```python
from build123d import *

# Parameters (mm, degrees)
F0_R     = 1.9812
F0_R_2   = 1.5
F0_R_3   = 1.3716
F0_W     = 4.99999
F0_H     = 51.988198
F0_W_2   = 17
F0_H_2   = 10.000005
F1_DEPTH = 2.999994


with BuildPart() as f1:
    # F0 (on Top) → F1 (new body)
    with BuildSketch(Plane.XY):
        with BuildLine():
            ThreePointArc((-161.572698, -117.981502), (-160.412138, -120.783342), (-157.610298, -121.943902))
            Line((-157.610298, -121.943902), (139.264902, -121.943902))
            Line((139.264902, -121.943902), (219.265302, -121.943902))
            ThreePointArc((219.265302, -121.943902), (222.066859, -120.783459), (223.227302, -117.981902))
            Line((223.227302, -117.981902), (223.227302, 117.807098))
            ThreePointArc((223.227302, 117.807098), (222.066859, 120.608655), (219.265302, 121.769098))
            Line((219.265302, 121.769098), (143.227302, 121.769098))
            Line((143.227302, 121.769098), (-9.640698, 121.769098))
            ThreePointArc((-9.640698, 121.769098), (-12.442255, 120.608655), (-13.602698, 117.807098))
            Line((-13.602698, 117.807098), (-13.602698, 113.769098))
            Line((-13.602698, 113.769098), (-18.621498, 113.769098))
            Line((-18.621498, 113.769098), (-18.621498, 111.609098))
            ThreePointArc((-18.621498, 111.609098), (-20.602698, 109.627898), (-22.583898, 111.609098))
            Line((-22.583898, 111.609098), (-22.583898, 113.769098))
            Line((-22.583898, 113.769098), (-143.081498, 113.769098))
            Line((-143.081498, 113.769098), (-143.081498, 111.609098))
            ThreePointArc((-143.081498, 111.609098), (-145.062698, 109.627898), (-147.043898, 111.609098))
            Line((-147.043898, 111.609098), (-147.043898, 113.769098))
            Line((-147.043898, 113.769098), (-157.610698, 113.769098))
            ThreePointArc((-157.610698, 113.769098), (-160.412255, 112.608655), (-161.572698, 109.807098))
            Line((-161.572698, 109.807098), (-161.572698, -117.981502))
        make_face()
        with Locations((-145.062698, -115.720902)):
            Circle(F0_R, mode=Mode.SUBTRACT)
        with Locations((-156.572698, -110.230902)):
            Circle(F0_R_2, mode=Mode.SUBTRACT)
        with Locations((-99.431735, -91.208814)):
            Circle(F0_R_3, mode=Mode.SUBTRACT)
        with Locations((-20.602698, -115.720902)):
            Circle(F0_R, mode=Mode.SUBTRACT)
        with Locations((30.427302, -110.230902)):
            Circle(F0_R_2, mode=Mode.SUBTRACT)
        with Locations((-50.435135, -91.208814)):
            Circle(F0_R_3, mode=Mode.SUBTRACT)
        with Locations((-43.882665, -62.214709)):
            Rectangle(F0_W, F0_H, mode=Mode.SUBTRACT)
        with Locations((20.768265, -91.208814)):
            Circle(F0_R_3, mode=Mode.SUBTRACT)
        with Locations((-145.062698, -43.330902)):
            Circle(F0_R, mode=Mode.SUBTRACT)
        with Locations((-99.431735, -33.220614)):
            Circle(F0_R_3, mode=Mode.SUBTRACT)
        with Locations((-156.572698, -4.230902)):
            Circle(F0_R_2, mode=Mode.SUBTRACT)
        with Locations((-93.072694, -24.711481)):
            Rectangle(F0_W_2, F0_H_2, mode=Mode.SUBTRACT)
        with Locations((-50.435135, -33.220614)):
            Circle(F0_R_3, mode=Mode.SUBTRACT)
        with Locations((-20.602698, -43.330902)):
            Circle(F0_R, mode=Mode.SUBTRACT)
        with Locations((20.768265, -33.220614)):
            Circle(F0_R_3, mode=Mode.SUBTRACT)
        with Locations((27.127306, -24.711481)):
            Rectangle(F0_W_2, F0_H_2, mode=Mode.SUBTRACT)
        with Locations((-6.572698, -4.230902)):
            Circle(F0_R_2, mode=Mode.SUBTRACT)
        with Locations((69.764865, -91.208814)):
            Circle(F0_R_3, mode=Mode.SUBTRACT)
        with Locations((76.317335, -62.214709)):
            Rectangle(F0_W, F0_H, mode=Mode.SUBTRACT)
        with Locations((136.877302, -115.593902)):
            Circle(F0_R, mode=Mode.SUBTRACT)
        with Locations((213.877302, -115.593902)):
            Circle(F0_R, mode=Mode.SUBTRACT)
        with Locations((217.427302, -110.230902)):
            Circle(F0_R_2, mode=Mode.SUBTRACT)
        with Locations((140.968265, -91.208814)):
            Circle(F0_R_3, mode=Mode.SUBTRACT)
        with Locations((189.964865, -91.208814)):
            Circle(F0_R_3, mode=Mode.SUBTRACT)
        with Locations((196.517335, -62.214709)):
            Rectangle(F0_W, F0_H, mode=Mode.SUBTRACT)
        with Locations((69.764865, -33.220614)):
            Circle(F0_R_3, mode=Mode.SUBTRACT)
        with Locations((136.877302, -43.203902)):
            Circle(F0_R, mode=Mode.SUBTRACT)
        with Locations((140.968265, -33.220614)):
            Circle(F0_R_3, mode=Mode.SUBTRACT)
        with Locations((189.964865, -33.220614)):
            Circle(F0_R_3, mode=Mode.SUBTRACT)
        with Locations((213.877302, -43.203902)):
            Circle(F0_R, mode=Mode.SUBTRACT)
        with Locations((147.327306, -24.711481)):
            Rectangle(F0_W_2, F0_H_2, mode=Mode.SUBTRACT)
        with Locations((217.427302, -1.230902)):
            Circle(F0_R_2, mode=Mode.SUBTRACT)
        with Locations((-99.431735, 13.791186)):
            Circle(F0_R_3, mode=Mode.SUBTRACT)
        with Locations((-50.435135, 13.791186)):
            Circle(F0_R_3, mode=Mode.SUBTRACT)
        with Locations((20.768265, 13.791186)):
            Circle(F0_R_3, mode=Mode.SUBTRACT)
        with Locations((-43.882665, 42.785291)):
            Rectangle(F0_W, F0_H, mode=Mode.SUBTRACT)
        with Locations((-99.431735, 71.779386)):
            Circle(F0_R_3, mode=Mode.SUBTRACT)
        with Locations((-93.072694, 80.288519)):
            Rectangle(F0_W_2, F0_H_2, mode=Mode.SUBTRACT)
        with Locations((-156.572698, 101.769098)):
            Circle(F0_R_2, mode=Mode.SUBTRACT)
        with Locations((-50.435135, 71.779386)):
            Circle(F0_R_3, mode=Mode.SUBTRACT)
        with Locations((20.768265, 71.779386)):
            Circle(F0_R_3, mode=Mode.SUBTRACT)
        with Locations((27.127306, 80.288519)):
            Rectangle(F0_W_2, F0_H_2, mode=Mode.SUBTRACT)
        with Locations((-5.602698, 111.609098)):
            Circle(F0_R_2, mode=Mode.SUBTRACT)
        with Locations((69.764865, 13.791186)):
            Circle(F0_R_3, mode=Mode.SUBTRACT)
        with Locations((76.317335, 42.785291)):
            Rectangle(F0_W, F0_H, mode=Mode.SUBTRACT)
        with Locations((140.968265, 13.791186)):
            Circle(F0_R_3, mode=Mode.SUBTRACT)
        with Locations((189.964865, 13.791186)):
            Circle(F0_R_3, mode=Mode.SUBTRACT)
        with Locations((196.517335, 42.785291)):
            Rectangle(F0_W, F0_H, mode=Mode.SUBTRACT)
        with Locations((69.764865, 71.779386)):
            Circle(F0_R_3, mode=Mode.SUBTRACT)
        with Locations((140.968265, 71.779386)):
            Circle(F0_R_3, mode=Mode.SUBTRACT)
        with Locations((147.327306, 80.288519)):
            Rectangle(F0_W_2, F0_H_2, mode=Mode.SUBTRACT)
        with Locations((136.877302, 88.749098)):
            Circle(F0_R, mode=Mode.SUBTRACT)
        with Locations((189.964865, 71.779386)):
            Circle(F0_R_3, mode=Mode.SUBTRACT)
        with Locations((201.397302, 111.609098)):
            Circle(F0_R_2, mode=Mode.SUBTRACT)
        with Locations((213.877302, 115.419098)):
            Circle(F0_R, mode=Mode.SUBTRACT)
    extrude(amount=F1_DEPTH)


solid = f1.part
```
Here's how the part is built. I have some questions about the finished solid (model axes, mm). Give positions to 0.01 mm unless a question says otherwise; leave off trailing zeros. Loops run counter-clockwise (first coordinate to the right, second up) from the corner with the lowest first, then second, coordinate; pieces in that order, holes last. Notation, with made-up numbers: M 12.5,83 L 60.5,83 A22 cw 60.5,121 Z; hole C 11.25,83.25 d2. An arc over 180 degrees is marked long. Use one line per item in the form item = value. Start each with the question number.
Q1. Will this pin go through, and if not, where does the flat tip stop? pin 1 Ø1.5 at (x, z) = (-152.5, 1.5) entering from +Y.
Q2. I need wall thicknesses on line 1 along Y through (x, z) = (153.5, 2.5); line 2 along X through (y, z) = (80, 2.4); line 3 along Y through (x, z) = (-42, 2.85). Which ranges of each line are inside material? Lowest first, please.
Q3. If we section it at C-C (z = 1.6): State how many separate pieces and enclosed holes the cut face has, then the cut area to 3 significant figures.
Q4. If we section it at B-B (x = -73): Write out the boundary of the cut face in (y, z).
Q5. If we section it at A-A (y = 30.5): Write out the boundary of the cut face in (x, z).
Taken from the geometry:
q1.pin_1 = 113.77
q2.line_1 = -121.94 to -29.71, -19.71 to 75.29, 85.29 to 121.77
q2.line_2 = -161.57 to -101.57, -84.57 to 18.63, 35.63 to 138.83, 155.83 to 223.23
q2.line_3 = -121.94 to -88.21, -36.22 to 16.79, 68.78 to 113.77
q3.separate_pieces = 1
q3.enclosed_holes = 55
q3.area = 89,600 mm^2
q4.outline = M -121.94,0 L 113.77,0 L 113.77,3 L -121.94,3 Z
q5.outline = M -161.57,0 L -46.38,0 L -46.38,3 L -161.57,3 Z; M -41.38,0 L 73.82,0 L 73.82,3 L -41.38,3 Z; M 78.82,0 L 194.02,0 L 194.02,3 L 78.82,3 Z; M 199.02,0 L 223.23,0 L 223.23,3 L 199.02,3 Z
